```python
from build123d import *

# Parameters (mm, degrees)
F0_R     = 50.8
F0_R_2   = 44.45
F1_DEPTH = 123.825
F2_R     = 44.45
F3_DEPTH = 9.525
F4_R     = 3.17499


# Not quite as in the source:
# - a fillet or chamfer is up to 0.001 mm smaller than in the source, because OpenCascade refuses the exact size
# - a feature names something its author has since deleted; it is built from what else it names


with BuildPart() as f1:
    # F0 (on Top) → F1 (new body)
    with BuildSketch(Plane.XY):
        Circle(F0_R)
        Circle(F0_R_2, mode=Mode.SUBTRACT)
    extrude(amount=F1_DEPTH)

    # F2 (on Top) → F3 (join)
    with BuildSketch(Plane.XY):
        Circle(F2_R)
    extrude(amount=F3_DEPTH)

    # F4 (radius 3.175 in the source; OpenCascade refuses exactly that, so slightly less here)
    f4_edges = [f1.edges().sort_by_distance(p)[0] for p in [
        (-44.45, 0, 123.825),
        (-50.8, 0, 123.825),
    ]]
    fillet(f4_edges, radius=F4_R)


solid = f1.part
```
Design review of the part built by this model. Coordinates are the model's own, in mm. Give positions to 0.01 mm unless a question says otherwise; leave off trailing zeros. Order: outer loops, then holes, each group sorted by start corner. A loop starts at its lowest first (then second) coordinate and runs counter-clockwise, first axis right, second up. Notation, with made-up numbers: M -40,57 L -15,57 A20 cw -15,71 Z; hole C -21.5,-33.75 d9. An arc over 180 degrees is marked long. One line per question, with ' | ' between items. Start each with the question number.
Q1. For pin 1 Ø8 at (y, z) = (37.5, 95) entering from -X; pin 2 Ø1 at (x, z) = (24, 56) entering from +Y; pin 3 Ø1 at (y, z) = (-26, 27) entering from +X, all flat-tipped, find the tip position at first contact; note any pin that passes through.
Q2. For L1, parallel to Y at x = 0, z = 56; L2, parallel to X at y = -1, z = 10; L3, parallel to Z at x = -15, y = -14 (3 decimals), list the stretches that pass through material, from the lowest coordinate up. Write a range as [from, to].
Q3. We need section B-B (z = 59.5). Write out the cut boundary in (x, y), plus the area to 3 significant figures.
Q4. The part is to be moulded in two halves that separate along X. For faces 1 (the face through (-1, 1, 0)), 2 (the face through (-11.012, -49.592, 59.48)), 3 (the face through (42.397, 13.352, 64.31)), say which applies: +X half, -X half, draft (parallel to the pull), parting line (faces both ways), or undercut.
Returned:
1) pin 1: x = -38.19 | pin 2: y = 45.04 | pin 3: x = 43.94
2) L1: [-50.8, -44.45], [44.45, 50.8] | L2: [-50.79, -44.44], [44.44, 50.79] | L3: [0, 9.525]
3) outline: C 0,0 d101.6; hole C 0,0 d88.9 | area: 1,900 mm2
4) face 1: draft | face 2: parting line | face 3: undercut
